from build123d import *

# Parameters (mm, degrees)
BOSS_EXTRUDE1_DEPTH = 171
SKETCH2_R           = 1.25
CUT_EXTRUDE1_DEPTH  = 10
SKETCH4_R           = 1.25
CUT_EXTRUDE2_DEPTH  = 10
LPATTERN1_COUNT     = 7
LPATTERN1_PITCH     = 25.5
SKETCH5_W           = 6
SKETCH5_H           = 6
CUT_EXTRUDE3_DEPTH  = 10
LPATTERN2_COUNT     = 19
LPATTERN2_PITCH     = 9
SKETCH6_W           = 39.406826709
SKETCH6_H           = 10.111121127
CUT_EXTRUDE4_DEPTH  = 36


with BuildPart() as part:
    # Sketch1 → Boss-Extrude1 (new body)
    with BuildSketch(Plane.XY):
        Polygon((-7.560747901, -2.297203345), (8.76644945, -1.788652997), (9.457807768, -2.612581756), (12.482904169, -0.866041535), (13.082904169, -1.905272019), (9.185789852, -4.155272019), (8.221608437, -3.006205355), (-6.986662858, -3.479904024), (-8.845450789, -5.695121219), (-12.742565106, -3.445121219), (-12.142565106, -2.405890734), (-9.117468705, -4.152430955), align=None)
    extrude(amount=BOSS_EXTRUDE1_DEPTH)

    # Sketch2 → Cut-Extrude1 (cut)
    with BuildSketch(Plane(origin=(3.495733027, -6.054787213, 0), x_dir=(0.8660254037844403, 0.49999999999999734, 0), z_dir=(-0.49999999999999734, 0.8660254037844403, 0))):
        with Locations(Location((8.377491356, -162, 0), (0, 0, 180))):
            Circle(SKETCH2_R)
    cut_extrude1 = extrude(amount=-CUT_EXTRUDE1_DEPTH, mode=Mode.SUBTRACT)

    # Sketch4 → Cut-Extrude2 (cut)
    with BuildSketch(Plane(origin=(-4.077422524, -7.062302975, 0), x_dir=(0.8660254037844392, -0.49999999999999917, 0), z_dir=(0.49999999999999917, 0.8660254037844392, 0))):
        with Locations(Location((-7.312824482, -162, 0), (0, 0, 180))):
            Circle(SKETCH4_R)
    cut_extrude2 = extrude(amount=-CUT_EXTRUDE2_DEPTH, mode=Mode.SUBTRACT)

    # LPattern1: Cut-Extrude1, Cut-Extrude2 ×7
    with Locations(*[(0, 0, -i * LPATTERN1_PITCH) for i in range(1, LPATTERN1_COUNT)]):
        add(cut_extrude1, mode=Mode.SUBTRACT)
        add(cut_extrude2, mode=Mode.SUBTRACT)

    # Sketch5 → Cut-Extrude3 (cut)
    with BuildSketch(Plane(origin=(0.064154599, -2.059707176, 0), x_dir=(0.9995152712604761, 0.031132338766899612, 0), z_dir=(-0.031132338766899612, 0.9995152712604761, 0))):
        with Locations((2.406515149, -166.5)):
            Rectangle(SKETCH5_W, SKETCH5_H)
    cut_extrude3 = extrude(amount=-CUT_EXTRUDE3_DEPTH, mode=Mode.SUBTRACT)

    # LPattern2: Cut-Extrude3 ×19
    with Locations(*[(0, 0, -i * LPATTERN2_PITCH) for i in range(1, LPATTERN2_COUNT)]):
        add(cut_extrude3, mode=Mode.SUBTRACT)

    # Sketch6 → Cut-Extrude4 (cut)
    with BuildSketch(Plane(origin=(0, 0, 0), x_dir=(-1, 0, 0), z_dir=(0, 0, -1))):
        with Locations((-0.40262443, -3.001999491)):
            Rectangle(SKETCH6_W, SKETCH6_H)
    extrude(amount=-CUT_EXTRUDE4_DEPTH, mode=Mode.SUBTRACT)


solid = part.part
For this review, take the finished solid that the model builds, in its own axes (mm). A direction names the side the tool comes from. Round coordinates to 2 decimals unless told otherwise and drop trailing zeros. Write each loop counter-clockwise with the first axis right and the second up, starting at its lowest first coordinate (ties: lowest second). Pieces come first, ordered by that corner, then holes. Notation, with made-up numbers: (58.5, 14.25) - (74.5, 14.25) arc R15 cw to (74.5, 30.25) - close; hole circle Ø1 at (-21.75, -36.75). An arc over 180 degrees is marked (long way). Use a Markdown table: item, result.
Q1. Wall thickness on line 1 along Z through (x, y) = (-10.5, -3.85); line 2 along X through (y, z) = (-2.5, 148); line 3 along X through (y, z) = (-3.75, 148.5): over which ranges is each line inside the solid? List them lowest first.
Derived:
| item | result |
|---|---|
| line 1 | z = 36 to 58.76, 61.24 to 84.26, 86.74 to 109.76, 112.24 to 135.26, 137.74 to 160.76, 163.24 to 171 |
| line 2 | x = -12.2 to -11.98, -7.73 to -0.52, 5.49 to 9.36, 9.65 to 12.05 |
| line 3 | x = -12.21 to -9.81, -8.78 to -7.21, 8.85 to 9.89 |
Q2. Machinability: for faces 5 (the flat face through (-10.767, -4.586, 102.555)), 6 (the flat face through (-10.651, -3.267, 102.555)), 7 (the flat face through (-7.9, -4.57, 102.56)), which of the approach directions +Z, -Z, +X, -X, +Y, -Y give a long, thin tool a straight path to every point of the face, cutting with its end or side? Answer none if there is none.
Derived:
| item | result |
|---|---|
| face 5 | +Z, -Z, -X, -Y |
| face 6 | +Z, -Z, +Y |
| face 7 | +Z, -Z, -Y |
Q3. We need section A-A (z = 144). Give the boundary of the cut face in (x, y).
Derived:
| item | result |
|---|---|
| outline | (-12.74, -3.45) - (-8.85, -5.7) - (-6.99, -3.48) - (8.22, -3.01) - (9.19, -4.16) - (13.08, -1.91) - (12.48, -0.87) - (9.46, -2.61) - (8.77, -1.79) - (-7.56, -2.3) - (-9.12, -4.15) - (-12.14, -2.41) - close |
Q4. Clearance check with flat-ended pins moving along their axes: pin 1 (10 mm diameter, centred on x = -1, z = 92.5, fed in from +Y); pin 2 (6 mm diameter, centred on x = 5.5, z = 72, fed in from -Y). State where each tip first meets the part, or that it passes through.
Derived:
| item | result |
|---|---|
| pin 1 | stops at y = -1.94 |
| pin 2 | stops at y = -3.34 |
Q5. The part is to be moulded in two halves that separate along Z. For faces 1 (the flat face through (0, -3, 36)), 2 (the cylindrical face through (-10.57, -4, 61.24)), 3 (the flat face through (10.95, -1.75, 102.56)), 4 (the flat face through (0, -3, 171)), say which applies: pulls with the +Z half, pulls with the -Z half, needs draft (parallel to the pull), parting line crosses it, or undercut.
Derived:
| item | result |
|---|---|
| face 1 | pulls with the -Z half |
| face 2 | undercut |
| face 3 | needs draft |
| face 4 | pulls with the +Z half |
